```python
from build123d import *

# Parameters (mm, degrees)
SKETCH_1_W          = 36
SKETCH_1_H          = 15
EXTRUDE_1_DEPTH     = 4
SKETCH_2_R          = 4
CUT_EXTRUDE_1_DEPTH = 20.906029237
SKETCH_4_R          = 1.5
CUT_EXTRUDE_2_DEPTH = 20.906029237
FILLET_1_R          = 3


with BuildPart() as part:
    # 草图1 → 凸台-拉伸1 (new body)
    with BuildSketch(Plane.XY):
        Rectangle(SKETCH_1_W, SKETCH_1_H)
    extrude(amount=EXTRUDE_1_DEPTH)

    # 草图2 → 切除-拉伸1 (cut, through all)
    with BuildSketch(Plane.XY.offset(4)):
        Circle(SKETCH_2_R)
    extrude(amount=-CUT_EXTRUDE_1_DEPTH, mode=Mode.SUBTRACT)

    # 草图4 → 切除-拉伸2 (cut, through all)
    with BuildSketch(Plane(origin=(0, 0, 0), x_dir=(-1, 0, 0), z_dir=(0, 0, -1))):
        with Locations((15, -3.5)):
            Circle(SKETCH_4_R)
        with Locations((15, 3.5)):
            Circle(SKETCH_4_R)
        with Locations((-15, 3.5)):
            Circle(SKETCH_4_R)
        with Locations((-15, -3.5)):
            Circle(SKETCH_4_R)
    extrude(amount=-CUT_EXTRUDE_2_DEPTH, mode=Mode.SUBTRACT)

    # 圆角1
    fillet_1_edges = [part.edges().sort_by_distance(p)[0] for p in [
        (-18, 7.5, 2),
        (18, 7.5, 2),
        (18, -7.5, 2),
        (-18, -7.5, 2),
    ]]
    fillet(fillet_1_edges, radius=FILLET_1_R)


solid = part.part
```
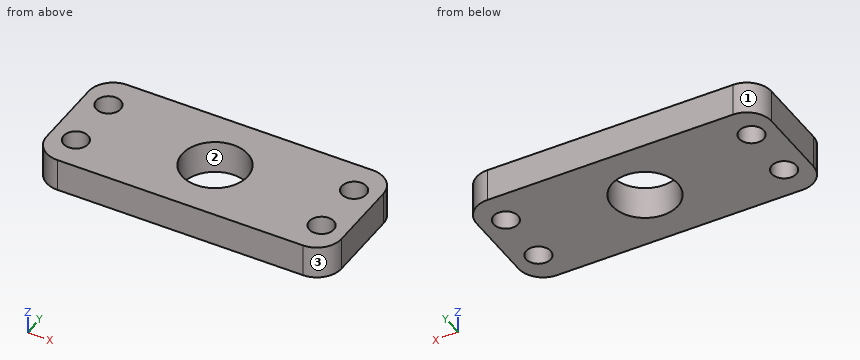
Input: part model. Units: mm. Frame: model coordinates. Face numbers are marked on the shaded views. Coordinates: 2 decimals unless noted, no trailing zeros. Loops run counter-clockwise (first coordinate to the right, second up) from the corner with the lowest first, then second, coordinate; pieces in that order, holes last. Notation, with made-up numbers: M 15,68.5 L 60,68.5 A7 cw 60,76.5 Z; hole C 42.25,83 d8. An arc over 180 degrees is marked long. One line per item, written item: value.
(1) Section B-B (x = 0). Output: boundary loops of the cut face in (y, z), and give its area (3 significant figures).
Filled in:
outline: M -7.5,0 L -4,0 L -4,4 L -7.5,4 Z; M 4,0 L 7.5,0 L 7.5,4 L 4,4 Z
area: 28.0 mm^2
(2) Section A-A (y = 0). Output: boundary loops of the cut face in (x, z), and give its area (3 significant figures).
Filled in:
outline: M -18,0 L -4,0 L -4,4 L -18,4 Z; M 4,0 L 18,0 L 18,4 L 4,4 Z
area: 112 mm^2
(3) Section D-D (y = 3.5). Output: boundary loops of the cut face in (x, z).
Filled in:
outline: M -18,0 L -16.5,0 L -16.5,4 L -18,4 Z; M -13.5,0 L -1.94,0 L -1.94,4 L -13.5,4 Z; M 1.94,0 L 13.5,0 L 13.5,4 L 1.94,4 Z; M 16.5,0 L 18,0 L 18,4 L 16.5,4 Z
(4) Line query: line 1 along Y through (x, z) = (15, 2.7); line 2 along X through (y, z) = (2.25, 3.35); line 3 along Y through (x, z) = (15.5, 0.25). Output: solid intervals per line, ascending. Write a range as from..to.
Filled in:
line 1: -7.5..-5, -2..2, 5..7.5
line 2: -18..-15.83, -14.17..-3.31, 3.31..14.17, 15.83..18
line 3: -7.46..-4.91, -2.09..2.09, 4.91..7.46
(5) Section C-C (z = 1.05). Output: boundary loops of the cut face in (x, y).
Filled in:
outline: M -18,-4.5 A3 ccw -15,-7.5 L 15,-7.5 A3 ccw 18,-4.5 L 18,4.5 A3 ccw 15,7.5 L -15,7.5 A3 ccw -18,4.5 Z; hole C -15,-3.5 d3; hole C -15,3.5 d3; hole C 0,0 d8; hole C 15,-3.5 d3; hole C 15,3.5 d3
(6) Pin query (flat end, axial travel): pin 1 (1.8 mm diameter, centred on x = -15, y = -3.5, fed in from -Z). Return the tip coordinate at first contact, or that it passes through.
Filled in:
pin 1: through
(7) Pull-direction query (Y, two-part tool) for the marked faces 1, 2 and 3; classes: +Y half, -Y half, draft (parallel to the pull), parting line (faces both ways), or undercut.
Filled in:
face 1: +Y half
face 2: undercut
face 3: -Y half
